```python
from build123d import *

# Parameters (mm, degrees)
PAD035_DEPTH    = 3
PAD036_DEPTH    = 10
SKETCH093_R     = 1.6
POCKET056_DEPTH = 5
SKETCH094_R     = 3.5
POCKET057_DEPTH = 3.5
SKETCH095_R     = 1.6
POCKET058_DEPTH = 10
SKETCH096_R     = 3.5
POCKET059_DEPTH = 6


with BuildPart() as part:
    # Sketch091 → Pad035 (new body)
    with BuildSketch(Plane.XY):
        with BuildLine():
            Line((-53, -7), (-35, -7))
            Line((-35, -7), (-35, 0))
            Line((-35, 0), (-27.91459, 0))
            Line((-27.91459, 0), (-27.91459, 25))
            Line((-27.91459, 25), (-44, 25))
            Line((-44, 23.115973), (-44, 25))
            ThreePointArc((-60, 23.115973), (-52, -3.477413), (-44, 23.115973))
            Line((-60, 23.115973), (-60, 25))
            Line((-60, 25), (-76.08541, 25))
            Line((-76.08541, 25), (-76.08541, 0))
            Line((-76.08541, 0), (-65.384759, 0))
            Line((-65.384759, 0), (-58, -7.384759))
            Line((-58, -7.384759), (-58, -25))
            Line((-58, -25), (-53, -25))
            Line((-53, -25), (-53, -7))
        make_face()
        with BuildLine():
            ThreePointArc((-71.6, 11), (-69.5, 8.9), (-67.4, 11))
            Line((-67.4, 11), (-67.4, 18))
            ThreePointArc((-67.4, 18), (-69.5, 20.1), (-71.6, 18))
            Line((-71.6, 11), (-71.6, 18))
        make_face(mode=Mode.SUBTRACT)
        with BuildLine():
            ThreePointArc((-36.6, 11), (-34.5, 8.9), (-32.4, 11))
            Line((-32.4, 11), (-32.4, 18))
            ThreePointArc((-32.4, 18), (-34.5, 20.1), (-36.6, 18))
            Line((-36.6, 11), (-36.6, 18))
        make_face(mode=Mode.SUBTRACT)
    extrude(amount=PAD035_DEPTH)

    # Sketch092 (on Face24 of Pad035) → Pad036 (join)
    with BuildSketch(Plane(origin=(0, 0, 0), x_dir=(1, 0, 0), z_dir=(0, 0, -1))):
        with BuildLine():
            Line((-53, 25), (-58, 25))
            Line((-58, 25), (-58, 7.384759))
            Line((-58, 7.384759), (-58, 2.564759))
            ThreePointArc((-41.98, 0), (-49.619239, 3.598228), (-58, 2.564759))
            Line((-41.98, 0), (-35, 0))
            Line((-35, 0), (-35, 7))
            Line((-35, 7), (-53, 7))
            Line((-53, 7), (-53, 25))
        make_face()
    extrude(amount=PAD036_DEPTH)

    # Sketch093 (on Face31 of Pad036) → Pocket056 (cut)
    with BuildSketch(Plane(origin=(-58, 0, 0), x_dir=(0, -1, 0), z_dir=(-1, 0, 0))):
        with Locations((17, -5)):
            Circle(SKETCH093_R)
    extrude(amount=-POCKET056_DEPTH, mode=Mode.SUBTRACT)

    # Sketch094 (on Face31 of Pocket056) → Pocket057 (cut)
    with BuildSketch(Plane(origin=(-58, 0, 0), x_dir=(0, -1, 0), z_dir=(-1, 0, 0))):
        with Locations((17, -5)):
            Circle(SKETCH094_R)
    extrude(amount=-POCKET057_DEPTH, mode=Mode.SUBTRACT)

    # Sketch095 (on Face11 of Pocket057) → Pocket058 (cut)
    with BuildSketch(Plane(origin=(0, 0, 0), x_dir=(-1, 0, 0), z_dir=(0, 1, 0))):
        with Locations((43, -5)):
            Circle(SKETCH095_R)
    extrude(amount=-POCKET058_DEPTH, mode=Mode.SUBTRACT)

    # Sketch096 (on Face11 of Pocket058) → Pocket059 (cut)
    with BuildSketch(Plane(origin=(0, 0, 0), x_dir=(-1, 0, 0), z_dir=(0, 1, 0))):
        with Locations((43, -5)):
            Circle(SKETCH096_R)
    extrude(amount=-POCKET059_DEPTH, mode=Mode.SUBTRACT)


with BuildPart() as part_1:
    # Body013 placement: moved
    add(part.part.moved(Location((0, 60, 110))))


solid = part_1.part
```
The model under review builds one solid part; all positions refer to its coordinate system, in mm. A direction names the side the tool comes from. Give positions to 0.01 mm unless a question says otherwise; leave off trailing zeros. Write each loop counter-clockwise with the first axis right and the second up, starting at its lowest first coordinate (ties: lowest second). Pieces come first, ordered by that corner, then holes. Notation, with made-up numbers: M 73,52.25 L 120,52.25 A33 ccw 120,87.25 Z; hole C 38.5,88.5 d6. An arc over 180 degrees is marked long. Write item = value, one per line. Start each with the question number.
Q1. We need section D-D (x = -52). State the section outline as (y, z) points, plus the area to 3 significant figures.
Q2. We need section B-B (z = 104.25). State the section outline as (x, y) points.
Q3. We need section C-C (y = 49). State the section outline as (x, z) points, plus the area to 3 significant figures.
Q4. Clearance check with flat-ended pins moving along their axes: pin 1 (6.5 mm diameter, centred on y = 43, z = 105, fed in from +X); pin 2 (10 mm diameter, centred on x = -42.5, y = 77, fed in from -Z); pin 3 (4 mm diameter, centred on y = 45, z = 108.5, fed in from -X); pin 4 (3 mm diameter, centred on x = -43, z = 105, fed in from -Y). State where each tip first meets the part, or that it passes through.
Q5. Mouldability with a two-part tool opening along Z and no side actions: class faces 6 (the face through (-53.4, 51.1, 100)), 7 (the face through (-54.5, 42, 103)), 8 (the face through (-61.744, 56.359, 111.479)) as released by +Z, released by -Z, zero draft, split by the parting line, or undercut.
Q6. Machinability: for faces 1 (the face through (-34.5, 80.1, 111.5)), 2 (the face through (-71, 60, 111)), 3 (the face through (-58, 46, 108)), 4 (the face through (-32, 60, 111)), 5 (the face through (-38, 60, 105)), which of the approach directions +Z, -Z, +X, -X, +Y, -Y give a long, thin tool a straight path to every point of the face, cutting with its end or side? Answer none if there is none.
Q7. For line 1 (X direction, y = 55.5, z = 105); line 2 (X direction, y = 53.2, z = 105); line 3 (Z direction, x = -43, y = 56.25), list the stretches that pass through material, from the lowest coordinate up.
Q8. We need section A-A (x = -69.5). State the section outline as (y, z) points, plus the area to 3 significant figures.
Result set:
q1.outline = M 53,100 L 56.21,100 L 56.21,110 L 56.52,110 L 56.52,113 L 53,113 Z
q1.area = 42.7 mm2
q2.outline = M -58,35 L -53,35 L -53,41.59 L -54.5,41.59 L -54.5,39.58 L -58,39.58 Z; M -58,46.42 L -54.5,46.42 L -54.5,44.41 L -53,44.41 L -53,53 L -44.41,53 L -44.41,54 L -46.42,54 L -46.42,57.28 A15.2 cw -58,57.44 Z; M -41.59,53 L -35,53 L -35,60 L -39.58,60 L -39.58,54 L -41.59,54 Z
q3.outline = M -58,100 L -53,100 L -53,113 L -58,113 Z
q3.area = 65.0 mm2
q4.pin_1 = -53
q4.pin_2 = 110
q4.pin_3 = -58
q4.pin_4 = through
q5.face_6 = released by -Z
q5.face_7 = undercut
q5.face_8 = zero draft
q6.face_1 = +Z, -Z
q6.face_2 = +Z, -Z, -X, -Y
q6.face_3 = -Z, -X, -Y
q6.face_4 = +Z, -Z, +X, -Y
q6.face_5 = -Z, +X, -X, +Y
q7.line_1 = -58 to -46.5, -39.5 to -35
q7.line_2 = -58 to -44.6, -41.4 to -35
q7.line_3 = 100 to 101.5, 108.5 to 113
q8.outline = M 60,110 L 68.9,110 L 68.9,113 L 60,113 Z; M 80.1,110 L 85,110 L 85,113 L 80.1,113 Z
q8.area = 41.4 mm2
